from build123d import *

# Parameters (mm, degrees)
SKETCH1_R         = 3.81
EXTRUDE1_DEPTH    = 17.78
SKETCH2_OUTSIDE_W = 13.778
SKETCH2_OUTSIDE_H = 13.778
SKETCH2_OUTSIDE_R = 2.4892
EXTRUDE2_DEPTH    = 12.7
EXTRUDE3_DEPTH    = 3.048


with BuildPart() as part:
    # Sketch1 → Extrude1 (new body)
    with BuildSketch(Plane.XY):
        Circle(SKETCH1_R)
    extrude(amount=EXTRUDE1_DEPTH)

    # Sketch2 outside → Extrude2 (cut)
    with BuildSketch(Plane.XY.offset(17.78)):
        Rectangle(SKETCH2_OUTSIDE_W, SKETCH2_OUTSIDE_H)
        Circle(SKETCH2_OUTSIDE_R, mode=Mode.SUBTRACT)
    extrude(amount=-EXTRUDE2_DEPTH, mode=Mode.SUBTRACT)

    # Sketch3 → Extrude3 (cut)
    with BuildSketch(Plane(origin=(0, 0, 0), x_dir=(-1, 0, 0), z_dir=(0, 0, -1))):
        Polygon((0, 2.987683948), (-2.587410198, 1.493841974), (-2.587410198, -1.493841974), (0, -2.987683948), (2.587410198, -1.493841974), (2.587410198, 1.493841974), align=None)
    extrude(amount=-EXTRUDE3_DEPTH, mode=Mode.SUBTRACT)


solid = part.part
Model file for the job. Use its own axes, mm. A direction names the side the tool comes from. Give positions to 0.01 mm unless a question says otherwise; leave off trailing zeros. Loops run counter-clockwise (first coordinate to the right, second up) from the corner with the lowest first, then second, coordinate; pieces in that order, holes last. Notation, with made-up numbers: (64.5, 35.25) - (105.5, 35.25) arc R22 cw to (105.5, 61.25) - close; hole circle Ø11 at (-5.5, 41). An arc over 180 degrees is marked (long way). Use one line per item in the form item = value.
(1) Cut at B-B (x = 0.75). Give the cut face in (y, z).
Determined:
outline = (-3.74, 0) - (-2.55, 0) - (-2.55, 3.05) - (2.55, 3.05) - (2.55, 0) - (3.74, 0) - (3.74, 5.08) - (2.37, 5.08) - (2.37, 17.78) - (-2.37, 17.78) - (-2.37, 5.08) - (-3.74, 5.08) - close
(2) Cut at A-A (y = 0). Give the cut face in (x, z).
Determined:
outline = (-3.81, 0) - (-2.59, 0) - (-2.59, 3.05) - (2.59, 3.05) - (2.59, 0) - (3.81, 0) - (3.81, 5.08) - (2.49, 5.08) - (2.49, 17.78) - (-2.49, 17.78) - (-2.49, 5.08) - (-3.81, 5.08) - close
(3) Drop flat-ended pins along their axis: P1, Ø2, axis at x = -1.5, y = 0.5, coming from the -Z side; P2, Ø1, axis at y = 0.5, z = 13, coming from the +X side. Give the stop position or say it passes through.
Determined:
P1 = 3.05
P2 = 2.49
(4) Cut at C-C (z = 7.75). Give the cut face in (x, y).
Determined:
outline = circle Ø4.98 at (0, 0)
(5) Cut at D-D (y = 2.75). Give the cut face in (x, z), then the cut area to 3 significant figures.
Determined:
outline = (-2.64, 0) - (-0.41, 0) - (-0.41, 3.05) - (0.41, 3.05) - (0.41, 0) - (2.64, 0) - (2.64, 5.08) - (-2.64, 5.08) - close
area = 24.3 mm^2
(6) Pull direction X, two halves, no side cores. Call faces 1 (the face through (-0.9, -2.5, 5.08)), 2 (the face through (1.31, -2.23, 1.5)), 3 (the face through (-0.83, -3.72, 2.5)): pulls with the +X half, pulls with the -X half, needs draft (parallel to the pull), parting line crosses it, or undercut.
Determined:
face_1 = needs draft
face_2 = undercut
face_3 = parting line crosses it
(7) Drill centre lines: L1, parallel to Z at x = -2.5, y = 1.5; L2, parallel to Z at x = -0.75, y = -1; L3, parallel to Y at x = 0, z = 8. Where is each one in solid material? Low to high.
Determined:
L1 = 3.05 to 5.08
L2 = 3.05 to 17.78
L3 = -2.49 to 2.49
(8) 3-axis set-ups, long thin cutter, end or side, ignore diameter. For faces 4 (the face through (0, 0, 17.78)), 5 (the face through (-2.587, 0, 2)), 6 (the face through (2.374, 0.748, 11.519)): which of +Z, -Z, +X, -X, +Y, -Y reach the whole face in a straight line?
Determined:
face_4 = +Z, +X, -X, +Y, -Y
face_5 = -Z
face_6 = +Z
